```python
from build123d import *

# Parameters (mm, degrees)
PAD_DEPTH       = 2.03
SKETCH001_R     = 1.65
POCKET_DEPTH    = 5
SKETCH002_W     = 6
SKETCH002_H     = 30
POCKET001_DEPTH = 5
SKETCH004_R     = 2
POCKET002_DEPTH = 5


with BuildPart() as part:
    # Sketch → Pad (new body)
    with BuildSketch(Plane.XY):
        with BuildLine():
            Line((5, 475), (160, 475))
            ThreePointArc((165, 470), (163.535534, 473.535534), (160, 475))
            Line((165, 470), (165, 5))
            ThreePointArc((160, 0), (163.535534, 1.464466), (165, 5))
            Line((160, 0), (5, 0))
            ThreePointArc((0, 5), (1.464466, 1.464466), (5, 0))
            Line((0, 5), (0, 470))
            ThreePointArc((5, 475), (1.464466, 473.535534), (0, 470))
        make_face()
    extrude(amount=PAD_DEPTH)

    # Sketch001 → Pocket (cut)
    with BuildSketch(Plane.XY.offset(2.03)):
        with Locations((137.5, 3.5)):
            Circle(SKETCH001_R)
        with Locations((27.5, 3.5)):
            Circle(SKETCH001_R)
        with Locations((82.5, 3.5)):
            Circle(SKETCH001_R)
        with Locations((3.5, 27.5)):
            Circle(SKETCH001_R)
        with Locations((161.5, 27.5)):
            Circle(SKETCH001_R)
        with Locations((161.5, 167.5)):
            Circle(SKETCH001_R)
        with Locations((161.5, 307.5)):
            Circle(SKETCH001_R)
        with Locations((3.5, 307.5)):
            Circle(SKETCH001_R)
        with Locations((3.5, 167.5)):
            Circle(SKETCH001_R)
        with Locations((3.5, 447.5)):
            Circle(SKETCH001_R)
        with Locations((27.5, 471.5)):
            Circle(SKETCH001_R)
        with Locations((82.5, 471.5)):
            Circle(SKETCH001_R)
        with Locations((137.5, 471.5)):
            Circle(SKETCH001_R)
        with Locations((161.5, 447.5)):
            Circle(SKETCH001_R)
    extrude(amount=-POCKET_DEPTH, mode=Mode.SUBTRACT)

    # Sketch002 → Pocket001 (cut)
    with BuildSketch(Plane.XY.offset(2.03)):
        with Locations((143.5, 426.5)):
            Rectangle(SKETCH002_W, SKETCH002_H)
    extrude(amount=-POCKET001_DEPTH, mode=Mode.SUBTRACT)

    # Sketch004 → Pocket002 (cut)
    with BuildSketch(Plane.XY.offset(2.03)):
        with Locations((118, 97.5)):
            Circle(SKETCH004_R)
        with Locations((118, 55.675)):
            Circle(SKETCH004_R)
        with Locations((52, 52.5)):
            Circle(SKETCH004_R)
        with Locations((52, 101.5)):
            Circle(SKETCH004_R)
        with Locations((110, 101.5)):
            Circle(SKETCH004_R)
        with Locations((110, 52.5)):
            Circle(SKETCH004_R)
    extrude(amount=-POCKET002_DEPTH, mode=Mode.SUBTRACT)


solid = part.part
```
CAD build for the part. Positions are in the model's coordinates, mm. Round coordinates to 2 decimals unless told otherwise and drop trailing zeros. Return JSON: item names as keys, results as strings. Group by question number.
Item 1: Flat gauge pin, fed straight in: pin 1 Ø2.5 at (x, y) = (161.5, 27.5) entering from -Z. Where does the tip first touch, or does it go through?
Item 2: Probe probe 1 along Y at (x, z) = (110, 1.5); probe 2 along Y at (x, z) = (138, 0.4); probe 3 along Y at (x, z) = (161.5, 0.8). List the from-to ranges inside material, lowest first.
Item 3: Mould opens along Z. For faces 1 (the face through (84, 241, 2.03)), 2 (the face through (84, 241, 0)) say: +Z half, -Z half, draft (parallel to the pull), parting line (faces both ways), or undercut.
Resolved:
{
 "1": {"pin 1": "passes through"},
 "2": {"probe 1": "y = 0 to 50.5, 54.5 to 99.5, 103.5 to 475", "probe 2": "y = 0 to 1.93, 5.07 to 469.93, 473.07 to 475", "probe 3": "y = 0.23 to 25.85, 29.15 to 165.85, 169.15 to 305.85, 309.15 to 445.85, 449.15 to 474.77"},
 "3": {"face 1": "+Z half", "face 2": "-Z half"}
}
